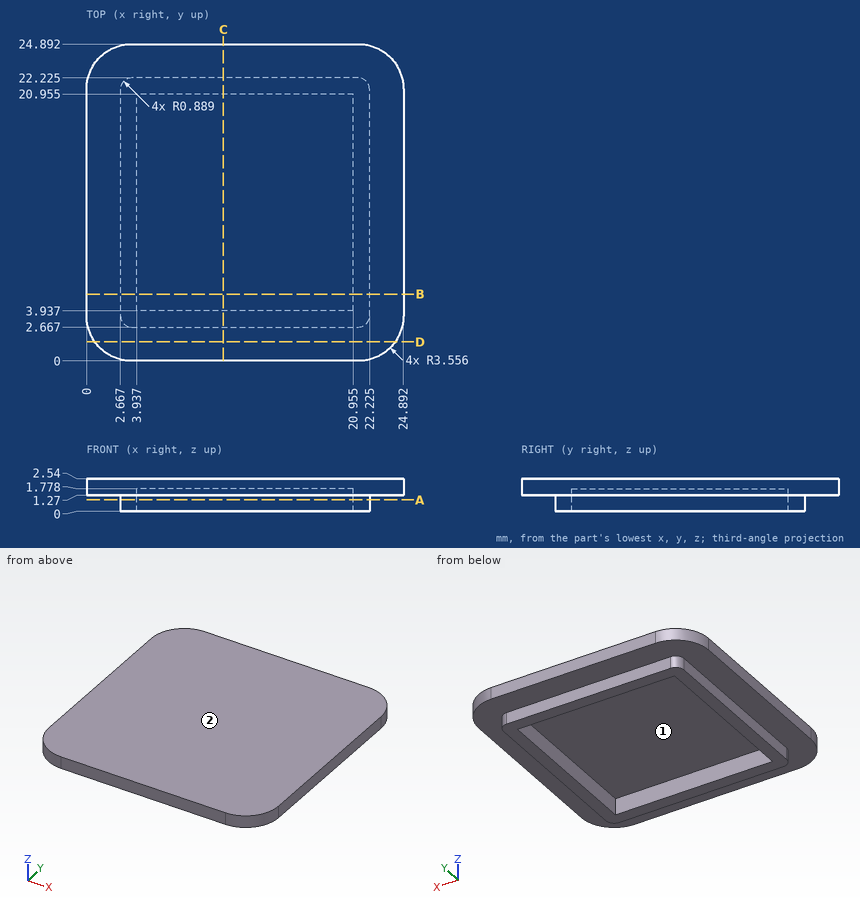
Design review of the part shown in the three views and the two pictorial views. Dimensions are in mm from the part's minimum x, y and z. Give positions to 0.01 mm unless a question says otherwise; leave off trailing zeros. Write each loop counter-clockwise with the first axis right and the second up, starting at its lowest first coordinate (ties: lowest second). Pieces come first, ordered by that corner, then holes. Notation, with made-up numbers: (-2, 23.5) - (47, 23.5) arc R10 ccw to (47, 29.5) - close; hole circle Ø4 at (71, 89). An arc over 180 degrees is marked (long way). Return JSON: item names as keys, results as strings. Group by question number.
(1) We need section B-B, the plane y = 5.25. Give the boundary of the cut face in (x, z) (3 decimals), then the cut area to 3 significant figures.
(2) Insertion check: pin 1 (10 mm diameter, centred on x = 15, y = 21, fed in from -Z); pin 2 (0.6 mm diameter, centred on y = 16.5, z = 0.5, fed in from -X); pin 3 (1.4 mm diameter, centred on y = 10, z = 0.5, fed in from +X) (3 decimals); pin 4 (5 mm diameter, centred on x = 12.5, y = 12.5, fed in from -Z). Each pin has a flat end and moves straight along its axis. Give the tip position at first contact, or say it passes through.
(3) We need section D-D, the plane y = 1.5. Give the boundary of the cut face in (x, z).
(4) To check wall thickness, follow probe 1 along Y at (x, z) = (7.75, 0.8) (3 decimals); probe 2 along X at (y, z) = (17.5, 1.3) (3 decimals). State the ranges of each line that lie inside material, in increasing order.
(5) We need section A-A, the plane z = 0.9. Give the boundary of the cut face in (x, y) (3 decimals).
(6) Mouldability with a two-part tool opening along Y and no side actions: class the marked faces 1 and 2 as +Y half, -Y half, draft (parallel to the pull), parting line (faces both ways), or undercut.
Reported:
{
 "1": {"outline": "(0, 1.27) - (2.667, 1.27) - (2.667, 0) - (3.937, 0) - (3.937, 1.778) - (20.955, 1.778) - (20.955, 0) - (22.225, 0) - (22.225, 1.27) - (24.892, 1.27) - (24.892, 2.54) - (0, 2.54) - close", "area": "26.2 mm2"},
 "2": {"pin 1": "stops at z = 0", "pin 2": "stops at x = 2.67", "pin 3": "stops at x = 22.225", "pin 4": "stops at z = 1.78"},
 "3": {"outline": "(0.65, 1.27) - (24.24, 1.27) - (24.24, 2.54) - (0.65, 2.54) - close"},
 "4": {"probe 1": "y = 2.667 to 3.937, 20.955 to 22.225", "probe 2": "x = 0 to 3.937, 20.955 to 24.892"},
 "5": {"outline": "(2.667, 3.556) arc R0.889 ccw to (3.556, 2.667) - (21.336, 2.667) arc R0.889 ccw to (22.225, 3.556) - (22.225, 21.336) arc R0.889 ccw to (21.336, 22.225) - (3.556, 22.225) arc R0.889 ccw to (2.667, 21.336) - close; hole (3.937, 3.937) - (20.955, 3.937) - (20.955, 20.955) - (3.937, 20.955) - close"},
 "6": {"face 1": "undercut", "face 2": "draft"}
}
